Could you check a few things on this drawing? It's one solid part, dimensions in mm from its lowest x, y, z. A direction names the side the tool comes from. Coordinates: 2 decimals unless noted, no trailing zeros. Write each loop counter-clockwise with the first axis right and the second up, starting at its lowest first coordinate (ties: lowest second). Pieces come first, ordered by that corner, then holes. Notation, with made-up numbers: M 16.5,23 L 36.5,23 A23 ccw 36.5,34 Z; hole C 6,38 d5. An arc over 180 degrees is marked long. Use a Markdown table: item, result.
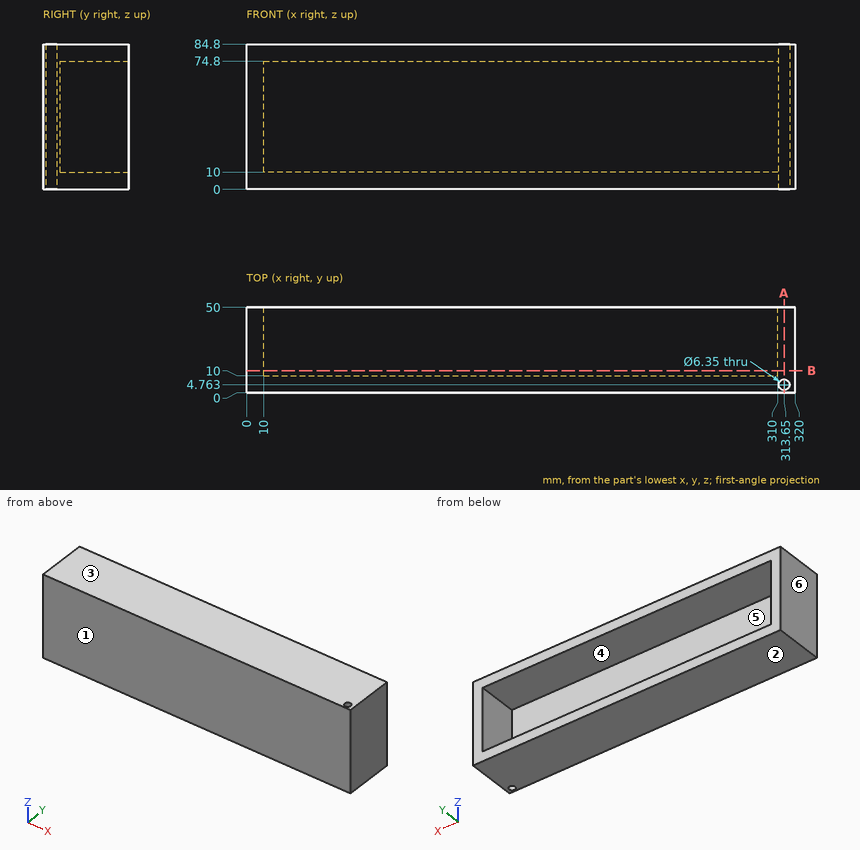
1. We'd pull the mould along Z, two halves only. Please class the marked faces 1, 2, 3 and 4: +Z half, -Z half, draft (parallel to the pull), parting line (faces both ways), or undercut.
Answers follow:
| item | result |
|---|---|
| face 1 | draft |
| face 2 | -Z half |
| face 3 | +Z half |
| face 4 | undercut |
2. I need wall thicknesses on probe 1 along X at (y, z) = (23, 45); probe 2 along Y at (x, z) = (313.65, 24); probe 3 along Z at (x, y) = (262, 26). Which ranges of each line are inside material? Lowest first, please.
Answers follow:
| item | result |
|---|---|
| probe 1 | x = 0 to 10, 310 to 320 |
| probe 2 | y = 0 to 1.59, 7.94 to 50 |
| probe 3 | z = 0 to 10, 74.8 to 84.8 |
3. Suppose I cut it at B-B on y = 13. Write out the boundary of the cut face in (x, z).
Answers follow:
| item | result |
|---|---|
| outline | M 0,0 L 320,0 L 320,84.8 L 0,84.8 Z; hole M 10,10 L 310,10 L 310,74.8 L 10,74.8 Z |
4. Which directions (+Z, -Z, +X, -X, +Y, -Y) give clear straight access to the entire face, cutting with the end or side of a thin tool? Please do the marked faces 5 and 6.
Answers follow:
| item | result |
|---|---|
| face 5 | +Y |
| face 6 | +Z, -Z, -X, +Y, -Y |
5. Suppose I cut it at A-A on x = 313.65. Write out the boundary of the cut face in (y, z).
Answers follow:
| item | result |
|---|---|
| outline | M 0,0 L 1.59,0 L 1.59,84.8 L 0,84.8 Z; M 7.94,0 L 50,0 L 50,84.8 L 7.94,84.8 Z |
